The model under review builds one solid part; all positions refer to its coordinate system, in mm. A direction names the side the tool comes from. Coordinates: 2 decimals unless noted, no trailing zeros. Order: outer loops, then holes, each group sorted by start corner. A loop starts at its lowest first (then second) coordinate and runs counter-clockwise, first axis right, second up. Notation, with made-up numbers: M 68,41 L 126,41 A25 cw 126,70 Z; hole C 48.5,24.25 d11. An arc over 180 degrees is marked long. One line per item, written item: value.
```python
from build123d import *

# Parameters (mm, degrees)
BOX001_W               = 10
BOX001_H               = 2
BOX001_DEPTH           = 2
BOX001_PLACEMENT_ANGLE = 20
BOX_W                  = 10
BOX_H                  = 2
BOX_DEPTH              = 2
BOX_PLACEMENT_ANGLE    = 20


with BuildPart() as cub001:
    # Box001 → Box001 (new body)
    with BuildSketch(Plane.XY):
        with Locations((5, 1)):
            Rectangle(BOX001_W, BOX001_H)
    extrude(amount=BOX001_DEPTH)


with BuildPart() as cub001_1:
    # Box001 placement: moved
    add(cub001.part.moved(Location((0.21404, 1.829385, 0))).rotate(Axis((0.21404, 1.829385, 0), (0, 0, -1)), BOX001_PLACEMENT_ANGLE))


with BuildPart() as fusion:
    # Box → Box (new body)
    with BuildSketch(Plane.XY):
        with Locations((5, 1)):
            Rectangle(BOX_W, BOX_H)
    extrude(amount=BOX_DEPTH)


with BuildPart() as fusion_1:
    # Box placement: moved
    add(fusion.part.moved(Location((0.985577, -1.589486, 0))).rotate(Axis((0.985577, -1.589486, 0), (0, 0, 1)), BOX_PLACEMENT_ANGLE))

    # Fusion: union Cub001
    add(cub001_1.part)


with BuildPart() as fusion_2:
    # Fusion placement: moved
    add(fusion_1.part.moved(Location((-5, -1, 0))))


solid = fusion_2.part
```
(1) For L1, parallel to Y at x = 4.5, z = 1.65; L2, parallel to Y at x = -2.25, z = 0.5; L3, parallel to Y at x = 0, z = 1.95, list the stretches that pass through material, from the lowest coordinate up.
Geometry results:
L1: y = -2.55 to -0.42, 0.51 to 2.64
L2: y = -1.95 to 2.03
L3: y = -1.13 to 1.22
(2) Mouldability with a two-part tool opening along X and no side actions: class faces 4 (the flat face through (2.47, 1.9, 0.99)), 5 (the flat face through (-4.449, 1.756, 0.986)), 6 (the flat face through (4.286, 0.432, 0.986)) as +X half, -X half, draft (parallel to the pull), parting line (faces both ways), or undercut.
Geometry results:
face 4: undercut
face 5: -X half
face 6: +X half
(3) We need section C-C, the plane x = 4.25. State the section outline as (y, z) points, plus the area to 3 significant figures.
Geometry results:
outline: M -2.46,0 L -0.33,0 L -0.33,2 L -2.46,2 Z; M 0.42,0 L 2.55,0 L 2.55,2 L 0.42,2 Z
area: 8.51 mm2
(4) Insertion check: pin 1 Ø1 at (y, z) = (2, 1.5) entering from -X; pin 2 Ø1 at (y, z) = (-1.5, 2) entering from +X. Each pin has a flat end and moves straight along its axis. Give the tip position at first contact, or say it passes through.
Geometry results:
pin 1: stops at x = -4.54
pin 2: stops at x = 5.19
(5) We need section A-A, the plane y = 1.4. State the section outline as (x, z) points, plus the area to 3 significant figures.
Geometry results:
outline: M -4.58,0 L -0.51,0 L -0.51,2 L -4.58,2 Z; M 1.1,0 L 5.18,0 L 5.18,2 L 1.1,2 Z
area: 16.3 mm2
(6) Tool access review of faces 1 (the flat face through (-1.889, -1.816, 0.986)), 2 (the flat face through (-3.72, 0.44, 0.99)), 3 (the flat face through (4.243, -0.329, 0.986)): name each direction out of +Z, -Z, +X, -X, +Y, -Y from which nothing blocks a thin tool from reaching the whole face with its end or side.
Geometry results:
face 1: +Z, -Z, -Y
face 2: +Z, -Z, -X
face 3: +Z, -Z, +X
(7) We need section B-B, the plane z = 0.35. State the section outline as (x, y) points (1 decimal), plus the area to 3 significant figures.
Geometry results:
outline: M -4.8,0.8 L -2.6,0 L -4.7,-0.7 L -4,-2.6 L 0.3,-1 L 4.6,-2.6 L 5.3,-0.7 L 3.2,0 L 5.4,0.8 L 4.7,2.7 L 0.3,1.1 L -4.1,2.7 Z
area: 33.8 mm2
(8) We need section D-D, the plane x = -0.5. State the section outline as (y, z) points.
Geometry results:
outline: M -1.31,0 L 1.4,0 L 1.4,2 L -1.31,2 Z
